Autodesk Inventor part; units mm, degrees
ref_plane "YZ Plane" through (0, 0, 0) normal (1, 0, 0) x (0, 1, 0)
ref_plane "XZ Plane" through (0, 0, 0) normal (0, 1, 0) x (-1, 0, 0)
ref_plane "XY Plane" through (0, 0, 0) normal (0, 0, 1) x (1, 0, 0)
sketch "Sketch1" plane through (0, 0, 0) normal (0, 1, 0) x (-1, 0, 0)
  line L0 (0, 0) -> (101.6, 0)
  line L1 (101.6, 0) -> (101.6, -152.4)
  line L2 (101.6, -152.4) -> (0, -152.4)
  line L3 (0, -152.4) -> (0, 0)
  dimension "d0" = 101.6
  dimension "d1" = 152.4
extrude "Extrusion1" add sketch "Sketch1" along normal blind 9.525
sketch "Sketch2" plane through (0, 9.525, 0) normal (0, 1, 0) x (1, 0, 0)
  line L0 (-101.6, 0) -> (0, 0)
  line L1 (0, 0) -> (-17.9605, 17.9605)
  line L2 (0, 0) -> (25.4, 0) construction
  line L3 (-101.6, 152.4) -> (-101.6, 0)
  line L4 (-101.6, 152.4) -> (-83.6395, 134.4395)
  line L5 (-17.9605, 17.9605) -> (-83.6395, 17.9605)
  line L6 (-83.6395, 17.9605) -> (-83.6395, 134.4395)
  line L7 (-83.6395, 134.4395) -> (-17.9605, 134.4395)
  line L8 (-17.9605, 134.4395) -> (-17.9605, 17.9605)
  dimension "d4" = 25.4
  dimension "d5" = 135
  dimension "d6" = 25.4
extrude "Extrusion2" cut sketch "Sketch2" against normal blind 9.525 contours L5 L6 L7 L8
sketch "Sketch3" plane through (0, 0, 0) normal (1, 0, 0) x (0, 0, -1)
  line L0 (0, 9.525) -> (152.4, 9.525)
  line L1 (0, 10.079) -> (25.4, 10.079) construction
  line L2 (0, 0) -> (0, 9.525)
  line L3 (0, 9.525) -> (23.8125, 9.525)
  line L4 (134.4395, 9.525) -> (17.9605, 9.525)
  circle A0 centre (23.8125, 9.525) radius 1.5875
  circle A1 centre (33.3375, 9.525) radius 1.5875
  circle A2 centre (42.8625, 9.525) radius 1.5875
  circle A3 centre (52.3875, 9.525) radius 1.5875
  circle A4 centre (61.9125, 9.525) radius 1.5875
  circle A5 centre (71.4375, 9.525) radius 1.5875
  circle A6 centre (80.9625, 9.525) radius 1.5875
  circle A7 centre (90.4875, 9.525) radius 1.5875
  circle A8 centre (100.0125, 9.525) radius 1.5875
  circle A9 centre (109.5375, 9.525) radius 1.5875
  circle A10 centre (119.0625, 9.525) radius 1.5875
  circle A11 centre (128.5875, 9.525) radius 1.5875
  point P0 (130.175, 9.525)
  point P1 (127, 9.525)
  point P2 (120.65, 9.525)
  point P3 (117.475, 9.525)
  point P4 (101.6, 9.525)
  point P5 (98.425, 9.525)
  point P6 (82.55, 9.525)
  point P7 (79.375, 9.525)
  point P8 (73.025, 9.525)
  point P9 (69.85, 9.525)
  point P10 (63.5, 9.525)
  point P11 (60.325, 9.525)
  point P12 (53.975, 9.525)
  point P13 (50.8, 9.525)
  point P14 (44.45, 9.525)
  point P15 (41.275, 9.525)
  point P16 (34.925, 9.525)
  point P17 (31.75, 9.525)
  point P18 (22.225, 9.525)
  point P19 (25.4, 9.525)
  dimension "d11" = 23.8125
  dimension "d12" = 3.175
  dimension "d15" = 9.525
extrude "Extrusion3" cut sketch "Sketch3" against normal blind 107.95 contours L0 A0 | L0 A11 | L0 A10 | A9 L0 | L0 A9 | L0 A8 | A7 L0 | L0 A7 | L0 A6 | L0 A5 | L0 A4 | L0 A3 | L0 A2 | L0 A1 picked at (24.8555, 9.3984) picked at (128.9035, 8.9629) picked at (119.4808, 8.612) picked at (100.4308, 8.612) picked at (81.3808, 8.612) picked at (71.8558, 8.612) picked at (61.501, 9.0475) picked at (52.5145, 8.7843) picked at (42.9895, 8.7843) picked at (33.5251, 8.5384)
sketch "Sketch4" plane through (0, 0, -152.4) normal (0, 0, -1) x (-1, 0, 0)
  line L0 (101.6, 0) -> (101.6, 9.525)
  line L1 (101.6, 4.7625) -> (67.7418, 4.7625)
  line L2 (0, 4.7625) -> (33.8582, 4.7625)
  line L3 (0, 4.7625) -> (33.8582, 4.7625) construction
  point P0 (0, 0)
  dimension "d22" = 33.8582
  dimension "d23" = 33.8582
  dimension "d24" = 0
hole "Hole1" at (-67.7418, 4.7625, -152.4) direction (0, 0, 1) diameter 4.9784 depth 25.4
hole "Hole2" at (-33.8582, 4.7625, -152.4) direction (0, 0, 1) diameter 4.9784 depth 25.4
sketch "Sketch5" plane through (0, 9.525, 0) normal (0, 1, 0) x (1, 0, 0)
  line L0 (-101.6, 0) -> (0, 0)
  line L1 (-50.8, 0) -> (-50.8, 17.9605)
  line L2 (-83.6395, 17.9605) -> (-17.9605, 17.9605)
  line L3 (-50.8, 0) -> (-50.8, 8.9803)
sketch "Sketch6" plane through (0, 9.525, 0) normal (0, 1, 0) x (1, 0, 0)
  line L0 (-17.9605, 134.4395) -> (-83.6395, 134.4395)
  line L1 (-50.8, 134.4395) -> (-50.8, 152.4)
  line L2 (0, 152.4) -> (-101.6, 152.4)
  line L3 (-50.8, 134.4395) -> (-50.8, 143.4197)
  point P0 (0, 0)
hole "Hole3" at (-50.8, 9.525, -8.9803) direction (0, -1, 0) diameter 4.9784 depth 25.4
hole "Hole4" at (-50.8, 9.525, -143.4197) direction (0, -1, 0) diameter 4.9784 depth 25.4
properties part number "side-A"
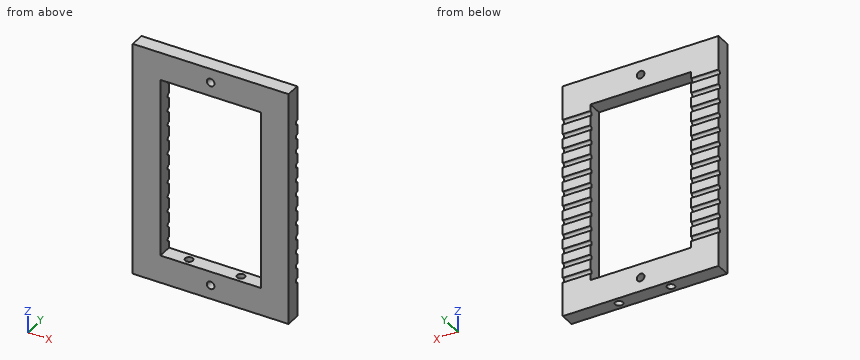
Check sheet for the modelled part. Datum: model origin and axes. Units: mm. Coordinates: 2 decimals unless noted, no trailing zeros. Order: outer loops, then holes, each group sorted by start corner. A loop starts at its lowest first (then second) coordinate and runs counter-clockwise, first axis right, second up. Notation, with made-up numbers: M 24,-15 L 55,-15 A24 ccw 55,4 Z; hole C 53.25,84.5 d9. An arc over 180 degrees is marked long. One line per question, with ' | ' between items. Start each with the question number.
Item 1: Gauge pin test, flat end, axial feed: P1, Ø3, axis at x = -50.8, z = -8.98, coming from the +Y side (1 decimal). Record the tip position at first contact, or that the pin passes through.
Item 2: Sectioned sample at C-C on x = -50.8. Record the cut outline in (y, z) (1 decimal), and give its area (3 significant figures).
Item 3: Sectioned sample at A-A on x = -80.5. Record the cut outline in (y, z) (1 decimal), and give its area (3 significant figures).
Item 4: Sectioned sample at B-B on y = 4.25. Record the cut outline in (x, z).
Item 5: Material ranges on line 1 (Z direction, x = -50.8, y = 6.75); line 2 (X direction, y = 2.5, z = -99.5); line 3 (Z direction, x = -24.5, y = 4.5), recorded low to high.
Answer below:
1) P1: passes through
2) outline: M 0,-152.4 L 9.5,-152.4 L 9.5,-145.9 L 0,-145.9 Z; M 0,-140.9 L 9.5,-140.9 L 9.5,-134.4 L 0,-134.4 Z; M 0,-18 L 9.5,-18 L 9.5,-11.5 L 0,-11.5 Z; M 0,-6.5 L 9.5,-6.5 L 9.5,0 L 0,0 Z | area: 247 mm^2
3) outline: M 0,-152.4 L 9.5,-152.4 L 9.5,-134.4 L 0,-134.4 Z; M 0,-18 L 9.5,-18 L 9.5,0 L 0,0 Z | area: 342 mm^2
4) outline: M -101.6,-152.4 L -70.18,-152.4 L -70.18,-134.44 L -83.64,-134.44 L -83.64,-17.96 L -17.96,-17.96 L -17.96,-134.44 L -31.42,-134.44 L -31.42,-152.4 L 0,-152.4 L 0,0 L -101.6,0 Z; M -65.31,-152.4 L -36.29,-152.4 L -36.29,-134.44 L -65.31,-134.44 Z; hole C -50.8,-143.42 d4.98; hole C -50.8,-8.98 d4.98
5) line 1: z = -152.4 to -145.91, -140.93 to -134.44, -17.96 to -11.47, -6.49 to 0 | line 2: x = -101.6 to -83.64, -17.96 to 0 | line 3: z = -152.4 to -134.44, -17.96 to 0
